Build history of the part. All positions in model axes, mm. A direction names the side the tool comes from. Give positions to 0.01 mm unless a question says otherwise; leave off trailing zeros. Write each loop counter-clockwise with the first axis right and the second up, starting at its lowest first coordinate (ties: lowest second). Pieces come first, ordered by that corner, then holes. Notation, with made-up numbers: (-20, 66) -> (-6, 66) arc R13 cw to (-6, 81) -> close; hole circle Ø11 at (27.25, -1). An arc over 180 degrees is marked (long way). Put each result on its own line as item: value.
Autodesk Inventor part; units mm, degrees
ref_plane "YZ Plane" through (0, 0, 0) normal (1, 0, 0) x (0, 1, 0)
ref_plane "XZ Plane" through (0, 0, 0) normal (0, 1, 0) x (-1, 0, 0)
ref_plane "XY Plane" through (0, 0, 0) normal (0, 0, 1) x (1, 0, 0)
sketch "Boceto1" plane through (0, 0, 0) normal (1, 0, 0) x (0, 1, 0)
  line L0 (-12.5, 15) -> (-12.5, 5)
  line L1 (-12.5, 5) -> (-15.5, 5)
  line L2 (-15.5, 5) -> (-15.5, -5)
  line L3 (-15.5, -5) -> (-12.5, -5)
  line L4 (-12.5, -5) -> (-12.5, -15)
  line L5 (-12.5, -15) -> (12.5, -15)
  line L6 (12.5, -15) -> (12.5, -5)
  line L7 (12.5, -5) -> (15.5, -5)
  line L8 (15.5, -5) -> (15.5, 5)
  line L9 (15.5, 5) -> (12.5, 5)
  line L10 (12.5, 5) -> (12.5, 15)
  line L11 (12.5, 15) -> (-12.5, 15)
  point P0 (0, 0)
extrude "Extrusión1" add sketch "Boceto1" along normal blind 3
properties part number "Battery_Wall1" material "MDF Tablero de fibras de densidad media"
1) Wall check: L1, parallel to Y at x = 1, z = -12.5. Give the ranges that are in metal, low to high.
Filled sheet:
L1: -12.5 to 12.5
2) Slice it at C-C (y = 13). Write the cut outline in (x, z), plus the area to 3 significant figures.
Filled sheet:
outline: (0, -5) -> (3, -5) -> (3, 5) -> (0, 5) -> close
area: 30.0 mm2
3) Slice it at B-B (z = 8). Write the cut outline in (x, y), plus the area to 3 significant figures.
Filled sheet:
outline: (0, -12.5) -> (3, -12.5) -> (3, 12.5) -> (0, 12.5) -> close
area: 75.0 mm2
4) Slice it at A-A (x = 0.8). Write the cut outline in (y, z), plus the area to 3 significant figures.
Filled sheet:
outline: (-15.5, -5) -> (-12.5, -5) -> (-12.5, -15) -> (12.5, -15) -> (12.5, -5) -> (15.5, -5) -> (15.5, 5) -> (12.5, 5) -> (12.5, 15) -> (-12.5, 15) -> (-12.5, 5) -> (-15.5, 5) -> close
area: 810 mm2
5) Tool access for faces 1 (the flat face through (1, 14, 5)), 2 (the flat face through (1, 14, -5)), 3 (the flat face through (1, -14, -5)), 4 (the flat face through (0, 0, 0)), 5 (the flat face through (1, -14, 5)): list every direction of +Z, -Z, +X, -X, +Y, -Y with a clear straight run to the whole face (end or side of a thin tool).
Filled sheet:
face 1: +Z, +X, -X, +Y
face 2: -Z, +X, -X, +Y
face 3: -Z, +X, -X, -Y
face 4: +Z, -Z, -X, +Y, -Y
face 5: +Z, +X, -X, -Y
6) Pin check, flat tips, straight feed: pin 1 (0.9 mm diameter, centred on x = 1, y = 14.5, fed in from -Z); pin 2 (1.5 mm diameter, centred on x = 1.5, z = 8, fed in from -Y). Stop position of each tip, or through.
Filled sheet:
pin 1: z = -5
pin 2: y = -12.5
